Source: CAD feature listing. Evaluate the final solid. Frame: model axes, mm. Round coordinates to 2 decimals unless told otherwise and drop trailing zeros. Write each loop counter-clockwise with the first axis right and the second up, starting at its lowest first coordinate (ties: lowest second). Pieces come first, ordered by that corner, then holes. Notation, with made-up numbers: M -23,14 L 29,14 A15 cw 29,24 Z; hole C 8.25,-34 d10. An arc over 180 degrees is marked long. Use a Markdown table: item, result.
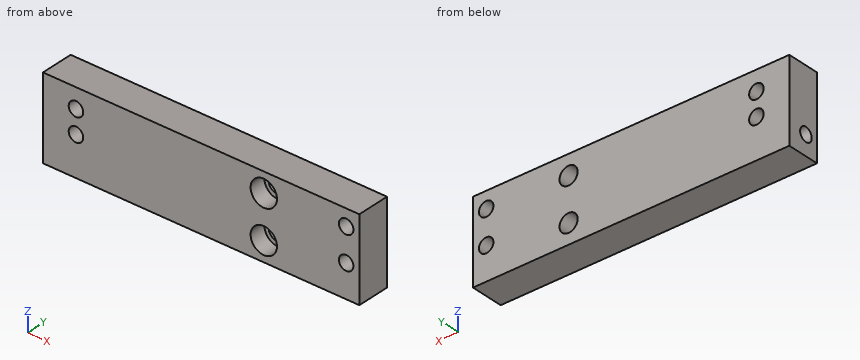
```python
from build123d import *

# Parameters (mm, degrees)
F0_W           = 96
F0_H           = 25
F1_DEPTH       = 10
F2_D           = 5.5
F2_CBORE_D     = 8
F2_CBORE_DEPTH = 5
F3_D           = 4.4
F5_D           = 4.2
F5_DEPTH       = 12
F5_TIP         = 1.2618073


with BuildPart() as f1:
    # F0 (on Front) → F1 (new body)
    with BuildSketch(Plane.XZ):
        Rectangle(F0_W, F0_H)
    extrude(amount=-F1_DEPTH)

    # F2 (through all)
    with Locations(Plane.XZ):
        with Locations((19, 6.5), (19, -6.5)):
            CounterBoreHole(F2_D / 2, F2_CBORE_D / 2, F2_CBORE_DEPTH)

    # F3 (through all)
    with Locations(Plane.XZ):
        with Locations((44, 7.5), (44, -2.5), (-38, 6.5), (-38, -0.5)):
            Hole(F3_D / 2)

    # F5
    with Locations(Plane(origin=(-48, 0, 0), x_dir=(0, -1, 0), z_dir=(-1, 0, 0))):
        with Locations((-4, -6.5)):
            Hole(F5_D / 2, depth=F5_DEPTH)
            with Locations((0, 0, -(F5_DEPTH + F5_TIP / 2))):  # 118° drill point
                Cone(0, F5_D / 2, F5_TIP, mode=Mode.SUBTRACT)


solid = f1.part
```
Q1. Line query: L1, parallel to Z at x = 44, y = 7; L2, parallel to Z at x = -38, y = 7.5; L3, parallel to Z at x = -39.5, y = 5. Output: solid intervals per line, ascending.
Results are:
| item | result |
|---|---|
| L1 | -12.5 to -4.7, -0.3 to 5.3, 9.7 to 12.5 |
| L2 | -12.5 to -2.7, 1.7 to 4.3, 8.7 to 12.5 |
| L3 | -12.5 to -8.35, -4.65 to -2.11, 1.11 to 4.89, 8.11 to 12.5 |
Q2. Section A-A on y = 7.5. Return loops of the section in (x, z), plus the area to 3 significant figures.
Results are:
| item | result |
|---|---|
| outline | M -48,-12.5 L 48,-12.5 L 48,12.5 L -48,12.5 Z; hole C -38,-0.5 d4.4; hole C -38,6.5 d4.4; hole C 19,-6.5 d5.5; hole C 19,6.5 d5.5; hole C 44,-2.5 d4.4; hole C 44,7.5 d4.4 |
| area | 2,290 mm^2 |
Q3. First-contact query: pin 1 Ø1 at (x, z) = (17.5, -9.5) entering from -Y; pin 2 Ø8 at (x, z) = (-5, -2.5) entering from -Y; pin 3 Ø4 at (y, z) = (4, -6.5) entering from -X; pin 4 Ø3.5 at (x, z) = (44, 7.5) entering from -Y. Flat tips, straight axial feed; report the tip coordinate or a pass-through.
Results are:
| item | result |
|---|---|
| pin 1 | y = 5 |
| pin 2 | y = 0 |
| pin 3 | x = -35.94 |
| pin 4 | through |
Q4. Section D-D on x = 19. Return loops of the section in (y, z), plus the area to 3 significant figures.
Results are:
| item | result |
|---|---|
| outline | M 0,-12.5 L 10,-12.5 L 10,-9.25 L 5,-9.25 L 5,-10.5 L 0,-10.5 Z; M 0,-2.5 L 5,-2.5 L 5,-3.75 L 10,-3.75 L 10,3.75 L 5,3.75 L 5,2.5 L 0,2.5 Z; M 0,10.5 L 5,10.5 L 5,9.25 L 10,9.25 L 10,12.5 L 0,12.5 Z |
| area | 115 mm^2 |
Q5. Section B-B on x = 44. Return loops of the section in (y, z).
Results are:
| item | result |
|---|---|
| outline | M 0,-12.5 L 10,-12.5 L 10,-4.7 L 0,-4.7 Z; M 0,-0.3 L 10,-0.3 L 10,5.3 L 0,5.3 Z; M 0,9.7 L 10,9.7 L 10,12.5 L 0,12.5 Z |
Q6. Section C-C on z = 7.5. Return loops of the section in (x, y), plus the area to 3 significant figures.
Results are:
| item | result |
|---|---|
| outline | M -48,0 L -39.96,0 L -39.96,10 L -48,10 Z; M -36.04,0 L 15.13,0 L 15.13,5 L 16.44,5 L 16.44,10 L -36.04,10 Z; M 21.56,5 L 22.87,5 L 22.87,0 L 41.8,0 L 41.8,10 L 21.56,10 Z; M 46.2,0 L 48,0 L 48,10 L 46.2,10 Z |
| area | 812 mm^2 |
